Design review of the part built by this model. Coordinates are the model's own, in mm. Coordinates: 2 decimals unless noted, no trailing zeros. Write each loop counter-clockwise with the first axis right and the second up, starting at its lowest first coordinate (ties: lowest second). Pieces come first, ordered by that corner, then holes.
Q1. Add section B-B, the plane y = 0. Give the boundary of the cut face in (x, z).
Q2. Add section C-C, the plane y = -52. Give the boundary of the cut face in (x, z), plus the area to 3 significant figures.
Q3. Add section D-D, the plane x = -53. Give the boundary of the cut face in (y, z), plus the area to 3 significant figures.
Q4. Add section A-A, the plane x = 0. Give the boundary of the cut face in (y, z).
Q5. To check wall thickness, follow probe 1 along Y at (x, z) = (0, 4.35); probe 2 along X at (y, z) = (24, 3.35); probe 3 along X at (y, z) = (45, 4.7). State the ranges of each line that lie inside material, in increasing order.
Q6. Clearance check with flat-ended pins moving along their axes: pin 1 Ø3.5 at (x, y) = (0, -52) entering from -Z; pin 2 Ø4.5 at (x, y) = (-29.5, -8) entering from -Z; pin 3 Ø2 at (x, z) = (10.5, 4.5) entering from -Y; pin 4 Ø2 at (y, z) = (-43.5, 2) entering from -X. State where each tip first meets the part, or that it passes through.
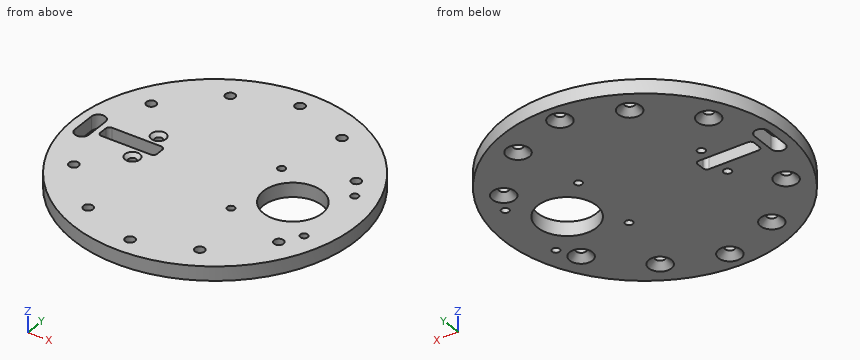
from build123d import *

# Parameters (mm, degrees)
SKETCH_R        = 1.65
SKETCH_W        = 24
SKETCH_H        = 6.4
PAD_DEPTH       = 6
CHAMFER_SIZE    = 2.75
CHAMFER001_SIZE = 1.5
FILLET_R        = 1.5


with BuildPart() as part:
    # Sketch → Pad (new body)
    with BuildSketch(Plane.XY):
        with BuildLine():
            ThreePointArc((60, 0), (0, 60), (-60, 0))
            ThreePointArc((-60, 0), (0, -60), (60, 0))
        make_face()
        with Locations((-29.5, 8)):
            Circle(SKETCH_R, mode=Mode.SUBTRACT)
        with Locations((-29.5, -8)):
            Circle(SKETCH_R, mode=Mode.SUBTRACT)
        with BuildLine():
            ThreePointArc((-2.05, -52), (0, -54.05), (2.05, -52))
            ThreePointArc((2.05, -52), (0, -49.95), (-2.05, -52))
        make_face(mode=Mode.SUBTRACT)
        with BuildLine():
            ThreePointArc((21.638077, -43.487067), (23.688077, -45.537067), (25.738077, -43.487067))
            ThreePointArc((25.738077, -43.487067), (23.688077, -41.437067), (21.638077, -43.487067))
        make_face(mode=Mode.SUBTRACT)
        with BuildLine():
            ThreePointArc((41.437067, -23.688077), (43.487067, -25.738077), (45.537067, -23.688077))
            ThreePointArc((45.537067, -23.688077), (43.487067, -21.638077), (41.437067, -23.688077))
        make_face(mode=Mode.SUBTRACT)
        with BuildLine():
            ThreePointArc((41.437067, 23.688077), (43.487067, 21.638077), (45.537067, 23.688077))
            ThreePointArc((45.537067, 23.688077), (43.487067, 25.738077), (41.437067, 23.688077))
        make_face(mode=Mode.SUBTRACT)
        with BuildLine():
            ThreePointArc((21.638077, 43.487067), (23.688077, 41.437067), (25.738077, 43.487067))
            ThreePointArc((25.738077, 43.487067), (23.688077, 45.537067), (21.638077, 43.487067))
        make_face(mode=Mode.SUBTRACT)
        with BuildLine():
            ThreePointArc((-2.05, 52), (0, 49.95), (2.05, 52))
            ThreePointArc((2.05, 52), (0, 54.05), (-2.05, 52))
        make_face(mode=Mode.SUBTRACT)
        with BuildLine():
            ThreePointArc((-25.738077, 43.487067), (-23.688077, 41.437067), (-21.638077, 43.487067))
            ThreePointArc((-21.638077, 43.487067), (-23.688077, 45.537067), (-25.738077, 43.487067))
        make_face(mode=Mode.SUBTRACT)
        with BuildLine():
            ThreePointArc((-45.537067, 23.688077), (-43.487067, 21.638077), (-41.437067, 23.688077))
            ThreePointArc((-41.437067, 23.688077), (-43.487067, 25.738077), (-45.537067, 23.688077))
        make_face(mode=Mode.SUBTRACT)
        with BuildLine():
            ThreePointArc((-45.537067, -23.688077), (-43.487067, -25.738077), (-41.437067, -23.688077))
            ThreePointArc((-41.437067, -23.688077), (-43.487067, -21.638077), (-45.537067, -23.688077))
        make_face(mode=Mode.SUBTRACT)
        with BuildLine():
            ThreePointArc((-25.738077, -43.487067), (-23.688077, -45.537067), (-21.638077, -43.487067))
            ThreePointArc((-21.638077, -43.487067), (-23.688077, -41.437067), (-25.738077, -43.487067))
        make_face(mode=Mode.SUBTRACT)
        with BuildLine():
            ThreePointArc((15.9, -15.5), (17.5, -17.1), (19.1, -15.5))
            ThreePointArc((19.1, -15.5), (17.5, -13.9), (15.9, -15.5))
        make_face(mode=Mode.SUBTRACT)
        with BuildLine():
            ThreePointArc((15.9, 15.5), (17.5, 13.9), (19.1, 15.5))
            ThreePointArc((19.1, 15.5), (17.5, 17.1), (15.9, 15.5))
        make_face(mode=Mode.SUBTRACT)
        with BuildLine():
            ThreePointArc((46.9, 15.5), (48.5, 13.9), (50.1, 15.5))
            ThreePointArc((50.1, 15.5), (48.5, 17.1), (46.9, 15.5))
        make_face(mode=Mode.SUBTRACT)
        with BuildLine():
            ThreePointArc((46.9, -15.5), (48.5, -17.1), (50.1, -15.5))
            ThreePointArc((50.1, -15.5), (48.5, -13.9), (46.9, -15.5))
        make_face(mode=Mode.SUBTRACT)
        with BuildLine():
            ThreePointArc((20.5, 0), (33, -12.5), (45.5, 0))
            ThreePointArc((45.5, 0), (33, 12.5), (20.5, 0))
        make_face(mode=Mode.SUBTRACT)
        with Locations((-35.5, 0)):
            Rectangle(SKETCH_W, SKETCH_H, mode=Mode.SUBTRACT)
        with BuildLine():
            ThreePointArc((-50, 5), (-53, 8), (-56, 5))
            Line((-56, 5), (-56, -5))
            ThreePointArc((-56, -5), (-53, -8), (-50, -5))
            Line((-50, 5), (-50, -5))
        make_face(mode=Mode.SUBTRACT)
    extrude(amount=PAD_DEPTH)

    # Chamfer
    chamfer_edges = [part.edges().sort_by_distance(p)[0] for p in [
        (43.487067, -25.738077, 0),
        (-43.487067, 21.638077, 0),
        (43.487067, 21.638077, 0),
        (0, 49.95, 0),
        (0, -54.05, 0),
        (23.688077, 41.437067, 0),
        (-43.487067, -25.738077, 0),
        (-23.688077, 41.437067, 0),
        (-23.688077, -45.537067, 0),
        (23.688077, -45.537067, 0),
    ]]
    chamfer(chamfer_edges, length=CHAMFER_SIZE)

    # Chamfer001
    chamfer001_edges = [part.edges().sort_by_distance(p)[0] for p in [
        (-31.15, -8, 6),
        (-31.15, 8, 6),
    ]]
    chamfer(chamfer001_edges, length=CHAMFER001_SIZE)

    # Fillet
    fillet_edges = [part.edges().sort_by_distance(p)[0] for p in [
        (-23.5, 3.2, 3),
        (-23.5, -3.2, 3),
        (-47.5, 3.2, 3),
        (-47.5, -3.2, 3),
    ]]
    fillet(fillet_edges, radius=FILLET_R)


solid = part.part
Here are the results:
1. outline: (-60, 0) - (-56, 0) - (-56, 6) - (-60, 6) - close; (-50, 0) - (-47.5, 0) - (-47.5, 6) - (-50, 6) - close; (-23.5, 0) - (20.5, 0) - (20.5, 6) - (-23.5, 6) - close; (45.5, 0) - (60, 0) - (60, 6) - (45.5, 6) - close
2. outline: (-29.93, 0) - (-4.8, 0) - (-2.05, 2.75) - (-2.05, 6) - (-29.93, 6) - close; (2.05, 2.75) - (4.8, 0) - (29.93, 0) - (29.93, 6) - (2.05, 6) - close
2. area: 327 mm2
3. outline: (-28.12, 0) - (-8, 0) - (-8, 6) - (-28.12, 6) - close; (8, 0) - (28.12, 0) - (28.12, 6) - (8, 6) - close
3. area: 241 mm2
4. outline: (-60, 0) - (-56.8, 0) - (-54.05, 2.75) - (-54.05, 6) - (-60, 6) - close; (-49.95, 2.75) - (-47.2, 0) - (47.2, 0) - (49.95, 2.75) - (49.95, 6) - (-49.95, 6) - close; (54.05, 2.75) - (56.8, 0) - (60, 0) - (60, 6) - (54.05, 6) - close
5. probe 1: y = -60 to -54.05, -49.95 to 49.95, 54.05 to 60
5. probe 2: x = -54.99 to -45.51, -41.46 to 41.46, 45.51 to 54.99
5. probe 3: x = -39.69 to -25.07, -22.3 to 22.3, 25.07 to 39.69
6. pin 1: passes through
6. pin 2: stops at z = 0
6. pin 3: stops at y = -59.24
6. pin 4: stops at x = -42.35
